Part print with two shaded views. Sizes in mm from the minimum x, y, z corner. Round coordinates to 2 decimals unless told otherwise and drop trailing zeros. Loops run counter-clockwise (first coordinate to the right, second up) from the corner with the lowest first, then second, coordinate; pieces in that order, holes last. Notation, with made-up numbers: (27.5, 63.5) -> (85.5, 63.5) arc R10 ccw to (85.5, 69.5) -> close; hole circle Ø7 at (31.5, 39.25). An arc over 180 degrees is marked (long way). Use a Markdown table: item, result. Add a question column.
Item 1: Flat gauge pin, fed straight in: pin 1 (3 mm diameter, centred on x = 235, y = 200, fed in from -Z). Where does the tip first touch, or does it go through?
Item 2: Probe line 1 (X direction, y = 200, z = 2.05); line 2 (X direction, y = 206.5, z = 2.85). List the from-to ranges inside material, lowest first. Write a range as [from, to].
Item 3: Cut at A-A, the plane y = 102. List the corners of the cut face in (x, z), plus the area to 3 significant figures.
Item 4: Cut at B-B, the plane z = 0.8. State how many separate pieces and enclosed holes the cut face has, plus the area to 3 significant figures.
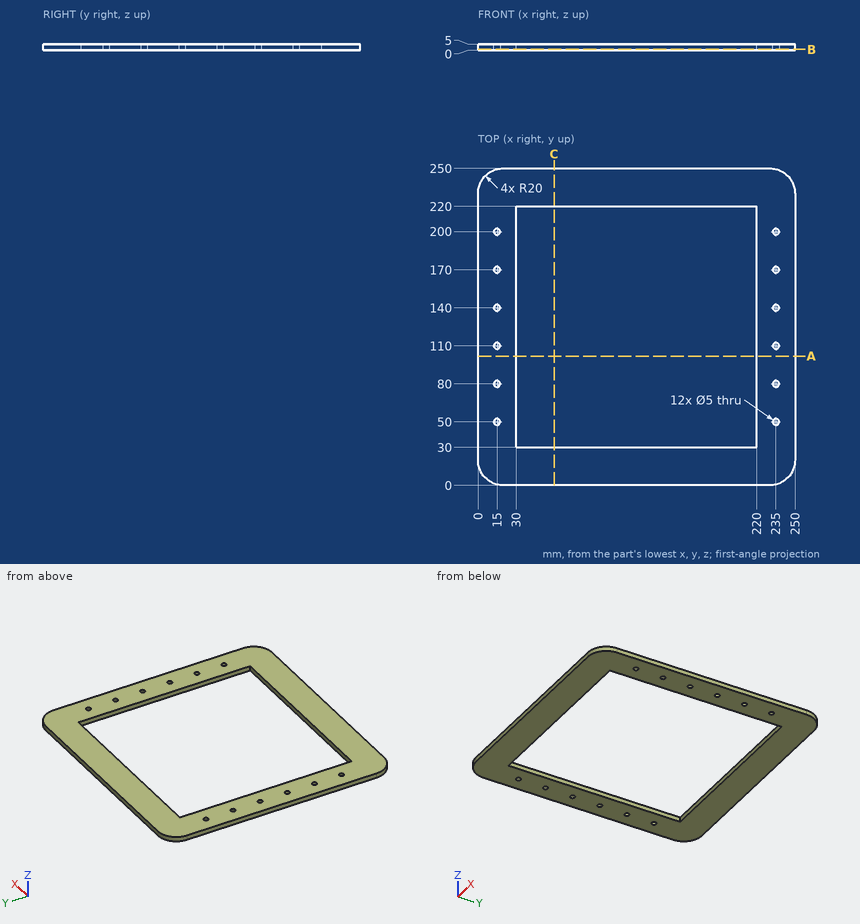
A:
| question | item | result |
|---|---|---|
| 1 | pin 1 | passes through |
| 2 | line 1 | x = [0, 12.5], [17.5, 30], [220, 232.5], [237.5, 250] |
| 2 | line 2 | x = [0, 30], [220, 250] |
| 3 | outline | (0, 0) -> (30, 0) -> (30, 5) -> (0, 5) -> close; (220, 0) -> (250, 0) -> (250, 5) -> (220, 5) -> close |
| 3 | area | 300 mm^2 |
| 4 | separate pieces | 1 |
| 4 | enclosed holes | 13 |
| 4 | area | 25,800 mm^2 |
